Job drawing, mm, ordinate dimensions from the low corner. One solid piece. Coordinates: 2 decimals unless noted, no trailing zeros. Order: outer loops, then holes, each group sorted by start corner. A loop starts at its lowest first (then second) coordinate and runs counter-clockwise, first axis right, second up. Notation, with made-up numbers: (-17, 84.5) - (35, 84.5) arc R7 cw to (35, 94.5) - close; hole circle Ø10 at (4, 56). An arc over 180 degrees is marked (long way). Write each question's results on one line, items separated by ' | '. Start each with the question number.
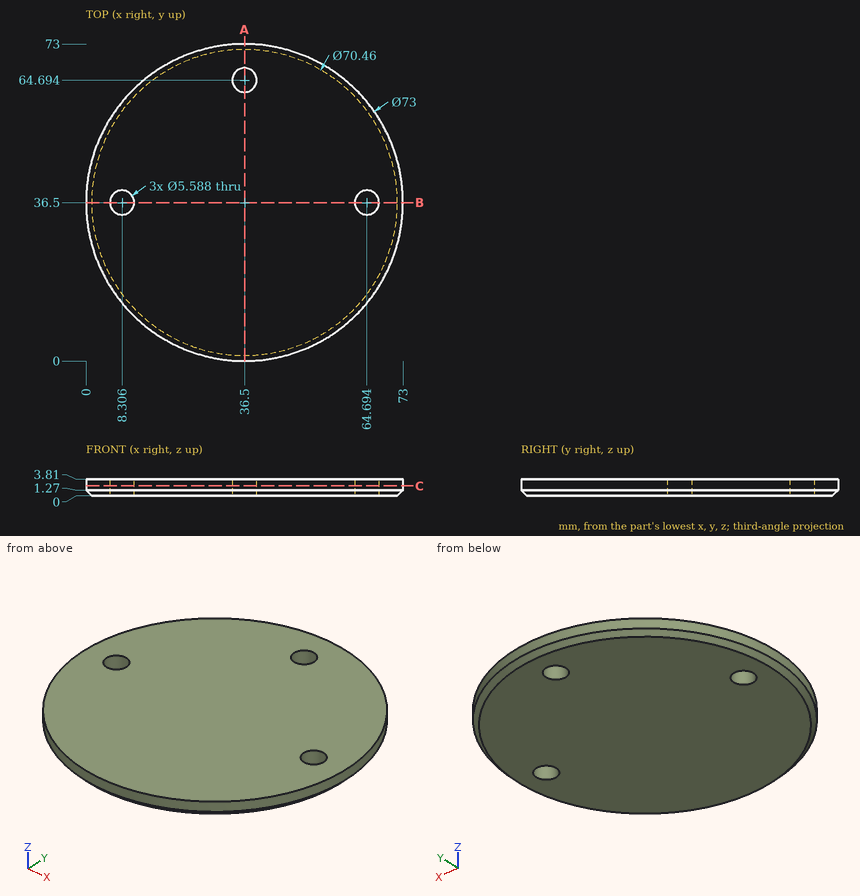
Item 1: Slice it at B-B (y = 36.5). Write the cut outline in (x, z).
Item 2: Probe probe 1 along Y at (x, z) = (36.5, 2.3); probe 2 along X at (y, z) = (38.5, 0.45) (3 decimals); probe 3 along Y at (x, z) = (37, 3.6). List the from-to ranges inside material, lowest first.
Item 3: Slice it at C-C (z = 2.2). Write the cut outline in (x, y).
Item 4: Slice it at A-A (x = 36.5). Write the cut outline in (y, z).
Item 5: Flat gauge pins, fed straight in: P1, Ø1.5, axis at x = 43.5, z = 1.5, coming from the -Y side; P2, Ø5, axis at x = 57.5, y = 7.5, coming from the -Z side; P3, Ø1, axis at y = 39.5, z = 3, coming from the +X side; P4, Ø1, axis at x = 54.5, z = 1, coming from the -Y side. Where does each tip first touch, or does it go through?
Resolved:
1) outline: (0, 1.27) - (1.27, 0) - (5.51, 0) - (5.51, 3.81) - (0, 3.81) - close; (11.1, 0) - (61.9, 0) - (61.9, 3.81) - (11.1, 3.81) - close; (67.49, 0) - (71.73, 0) - (73, 1.27) - (73, 3.81) - (67.49, 3.81) - close
2) probe 1: 0 to 61.9, 67.49 to 73 | probe 2: 0.876 to 6.355, 10.257 to 62.743, 66.645 to 72.124 | probe 3: 0 to 61.95, 67.44 to 73
3) outline: circle Ø73 at (36.5, 36.5); hole circle Ø5.59 at (8.31, 36.5); hole circle Ø5.59 at (36.5, 64.69); hole circle Ø5.59 at (64.69, 36.5)
4) outline: (0, 1.27) - (1.27, 0) - (61.9, 0) - (61.9, 3.81) - (0, 3.81) - close; (67.49, 0) - (71.73, 0) - (73, 1.27) - (73, 3.81) - (67.49, 3.81) - close
5) P1: y = 0.54 | P2: z = 0 | P3: x = 72.91 | P4: y = 4.51
